Input: part model. Units: mm. Frame: model coordinates. A direction names the side the tool comes from. Coordinates: 2 decimals unless noted, no trailing zeros. Order: outer loops, then holes, each group sorted by start corner. A loop starts at its lowest first (then second) coordinate and runs counter-clockwise, first axis right, second up. Notation, with made-up numbers: (46.5, 46) -> (53.5, 46) arc R28 cw to (53.5, 65) -> close; hole circle Ø9 at (14.5, -27.75). An arc over 180 degrees is marked (long way). One line per question, with ' | ' between items.
```python
from build123d import *

# Parameters (mm, degrees)
BOSS_EXTRUDE1_DEPTH             = 6.5
BOSS_EXTRUDE2_DEPTH             = 5.5
BOSS_EXTRUDE2_DEPTH_BACK        = 5.5
CUT_EXTRUDE1_START              = -4
CUT_EXTRUDE1_DEPTH              = 25
BOSS_EXTRUDE3_REACH             = 7.5
BOSS_EXTRUDE3_DIRECTION_2_REACH = 7.5
CUT_EXTRUDE2_DEPTH              = 4


with BuildPart() as part:
    # Sketch1 → Boss-Extrude1 (new body, symmetric)
    with BuildSketch(Plane.XY):
        with BuildLine():
            Line((-4, -0.75), (-4, 4.75))
            Line((-4, 4.75), (4, 4.75))
            Line((4, 4.75), (4, -0.75))
            ThreePointArc((4, -0.75), (0, -4.75), (-4, -0.75))
        make_face()
    extrude(amount=BOSS_EXTRUDE1_DEPTH, both=True)

    # Sketch2 → Boss-Extrude2 (add, two sides)
    with BuildSketch(Plane(origin=(0, 0, 0), x_dir=(0, 0, -1), z_dir=(1, 0, 0))) as boss_extrude2_sk:
        Polygon((-2.501037691, -0.25), (-0.059488514, -0.25), (2.39940586, 3.261665098), (3.441549178, 4.75), (1, 4.75), align=None)
        Polygon((4.591549178, 4.75), (4.021496439, 3.935880318), (3.690341929, 3.462942665), (1.090511486, -0.25), (3.532060664, -0.25), (7.033098355, 4.75), align=None)
    extrude(amount=BOSS_EXTRUDE2_DEPTH)
    extrude(boss_extrude2_sk.sketch, amount=-BOSS_EXTRUDE2_DEPTH_BACK)

    # Sketch3 → Cut-Extrude1 (cut)
    with BuildSketch(Plane.XY.offset(6.5).offset(CUT_EXTRUDE1_START)):
        with BuildLine():
            Line((4, -0.75), (3, -0.75))
            Line((3, -0.75), (3, 4.75))
            Line((3, 4.75), (-3, 4.75))
            Line((-3, 4.75), (-3, -0.75))
            Line((-3, -0.75), (-4, -0.75))
            ThreePointArc((-4, -0.75), (0, -4.75), (4, -0.75))
        make_face()
    extrude(amount=-CUT_EXTRUDE1_DEPTH, mode=Mode.SUBTRACT)

    # Boss-Extrude3: up to this face of the body (flat: up to its plane)
    boss_extrude3_end = Plane(part.part.faces().sort_by_distance((5.5, 2.25, -4.061804921))[0])
    # Sketch4 → Boss-Extrude3 (add, up to the picked face)
    with BuildSketch(Plane(origin=(0, 0, 0), x_dir=(0, 0, -1), z_dir=(1, 0, 0)), mode=Mode.PRIVATE) as boss_extrude3_sk1:
        Polygon((7.033098355, 4.75), (4.591549178, 4.75), (3.891341639, 3.75), (6.332890817, 3.75), align=None)
    boss_extrude3_tool1 = split(extrude(boss_extrude3_sk1.sketch, amount=BOSS_EXTRUDE3_REACH, mode=Mode.PRIVATE), bisect_by=boss_extrude3_end, keep=Keep.BOTH, mode=Mode.PRIVATE)
    add(boss_extrude3_tool1.solids().sort_by_distance((0, 4.25, -5.46222))[0])

    # Boss-Extrude3 direction 2: up to this face of the body (flat: up to its plane)
    boss_extrude3_direction_2_end = Plane(part.part.faces().sort_by_distance((-5.5, 2.25, -4.061804921))[0])
    # Sketch4 → Boss-Extrude3 direction 2 (add, up to the picked face)
    with BuildSketch(Plane(origin=(0, 0, 0), x_dir=(0, 0, -1), z_dir=(1, 0, 0)), mode=Mode.PRIVATE) as boss_extrude3_direction_2_sk1:
        Polygon((7.033098355, 4.75), (4.591549178, 4.75), (3.891341639, 3.75), (6.332890817, 3.75), align=None)
    boss_extrude3_direction_2_tool1 = split(extrude(boss_extrude3_direction_2_sk1.sketch, amount=-BOSS_EXTRUDE3_DIRECTION_2_REACH, mode=Mode.PRIVATE), bisect_by=boss_extrude3_direction_2_end, keep=Keep.BOTH, mode=Mode.PRIVATE)
    add(boss_extrude3_direction_2_tool1.solids().sort_by_distance((0, 4.25, -5.46222))[0])

    # Sketch5 → Cut-Extrude2 (cut)
    with BuildSketch(Plane.XY.offset(6.5)):
        Polygon((-0.6, 4.1), (-0.6, -4.1), (0.6, -4.1), (1.8, -3.25), (1.8, 3.25), (0.6, 4.1), align=None)
    extrude(amount=-CUT_EXTRUDE2_DEPTH, mode=Mode.SUBTRACT)


solid = part.part
```
1. Pin query (flat end, axial travel): pin 1 Ø1.1 at (x, y) = (-3.5, 2.5) entering from -Z; pin 2 Ø1 at (x, z) = (-1, 3) entering from -Y; pin 3 Ø1.1 at (x, z) = (-3.5, -4) entering from -Y; pin 4 Ø2 at (y, z) = (-2.5, 0.5) entering from -X. Return the tip coordinate at first contact, or that it passes through.
Recorded:
pin 1: stops at z = -6.5 | pin 2: stops at y = -4.72 | pin 3: stops at y = -0.75 | pin 4: passes through
2. Ray query, line 1 (X direction, y = 2.25, z = 3); line 2 (X direction, y = 0.5, z = -0.5); line 3 (Z direction, x = 3.25, y = 3.25). Return the intervals inside material, ascending. Write a range as [from, to].
Recorded:
line 1: x = [-4, -0.6], [1.8, 4] | line 2: x = [-4, -3], [3, 4] | line 3: z = [-6.5, 6.5]
3. Cut plane A-A, the plane x = 0. Return loops of the section in (y, z).
Recorded:
outline: (-4.75, 2.5) -> (-4.1, 2.5) -> (-4.1, 6.5) -> (-4.75, 6.5) -> close; (3.75, -6.33) -> (4.75, -7.03) -> (4.75, -4.59) -> (3.75, -3.89) -> close; (4.1, 2.5) -> (4.75, 2.5) -> (4.75, 6.5) -> (4.1, 6.5) -> close
4. Cut plane C-C, the plane z = 3.25. Return loops of the section in (x, y), and give its area (3 significant figures).
Recorded:
outline: (-4, -0.75) arc R4 ccw to (4, -0.75) -> (4, 4.75) -> (-4, 4.75) -> close; hole (-0.6, -4.1) -> (0.6, -4.1) -> (1.8, -3.25) -> (1.8, 3.25) -> (0.6, 4.1) -> (-0.6, 4.1) -> close | area: 50.5 mm^2
5. Cut plane D-D, the plane z = -3.25. Return loops of the section in (x, y).
Recorded:
outline: (-5.5, -0.25) -> (-4, -0.25) -> (-4, -0.75) -> (-3, -0.75) -> (-3, 4.75) -> (-5.5, 4.75) -> (-5.5, 4.48) -> (-4, 4.48) -> (-4, 2.83) -> (-5.5, 2.83) -> close; (3, -0.75) -> (4, -0.75) -> (4, -0.25) -> (5.5, -0.25) -> (5.5, 2.83) -> (4, 2.83) -> (4, 4.48) -> (5.5, 4.48) -> (5.5, 4.75) -> (3, 4.75) -> close
6. Cut plane B-B, the plane x = 4.5. Return loops of the section in (y, z).
Recorded:
outline: (-0.25, -3.53) -> (4.75, -7.03) -> (4.75, -4.59) -> (-0.25, -1.09) -> close; (-0.25, 0.06) -> (4.75, -3.44) -> (4.75, -1) -> (-0.25, 2.5) -> close
7. Access query for faces 4 (the face through (5, -0.25, -2)), 5 (the face through (-5, -0.25, 1)), 6 (the face through (-3.5, -0.75, -1.9)). Directions: +Z, -Z, +X, -X, +Y, -Y. A direction counts if a zero-diameter tool reaches every point of the face in a straight line with its end or side. Return the directions, or none.
Recorded:
face 4: +Z, -Z, +X, -Y | face 5: +Z, -Z, -X, -Y | face 6: -Z, +X, -X, -Y
8. Mould query, pull axis Z, two halves, no side actions, for faces 1 (the face through (3.5, 1.7, -6.5)), 2 (the face through (-5.5, 2, 0)), 3 (the face through (0.04, 4.26, -4.25)). Classes: released by +Z, released by -Z, zero draft, split by the parting line, or undercut.
Recorded:
face 1: released by -Z | face 2: zero draft | face 3: undercut
